The model under review builds one solid part; all positions refer to its coordinate system, in mm. A direction names the side the tool comes from. Give positions to 0.01 mm unless a question says otherwise; leave off trailing zeros. Write each loop counter-clockwise with the first axis right and the second up, starting at its lowest first coordinate (ties: lowest second). Pieces come first, ordered by that corner, then holes. Notation, with made-up numbers: (31.25, 89) - (71.25, 89) arc R19 ccw to (71.25, 123) - close; hole circle Ø5 at (34.5, 48.25). An arc over 180 degrees is marked (long way). Write item = value, one per line.
```python
from build123d import *

# Parameters (mm, degrees)
SKETCH1_W           = 171.45
SKETCH1_H           = 107.95
BOSS_EXTRUDE1_DEPTH = 3.175
BOSS_EXTRUDE2_DEPTH = 3.175
SKETCH4_W           = 50.8
SKETCH4_H           = 3.175
BOSS_EXTRUDE3_DEPTH = 19.05
CHAMFER1_SIZE       = 12.7
CHAMFER1_SIZE_2     = 10.472688289
CHAMFER1_SIZE_3     = 17.454480482
SKETCH6_W           = 88.9
SKETCH6_H           = 88.9
BOSS_EXTRUDE4_DEPTH = 3.175
BOSS_EXTRUDE7_DEPTH = 50.8


with BuildPart() as part:
    # Sketch1 → Boss-Extrude1 (new body)
    with BuildSketch(Plane(origin=(0, 0, 0), x_dir=(1, 0, 0), z_dir=(0, 1, 0))):
        Rectangle(SKETCH1_W, SKETCH1_H)
    extrude(amount=BOSS_EXTRUDE1_DEPTH)

    # Sketch2 → Boss-Extrude2 (add)
    with BuildSketch(Plane(origin=(0, 3.175, 0), x_dir=(1, 0, 0), z_dir=(0, 1, 0))):
        Polygon((-85.725, -53.975), (-82.55, -66.675), (88.9, -66.675), (85.725, -53.975), align=None)
    extrude(amount=-BOSS_EXTRUDE2_DEPTH)

    # Chamfer1
    # the kernel refuses this chamfer: 17.454480482, 12.7, 10.472688289 mm, written as the material it takes off along each edge
    with BuildSketch(Plane(origin=(88.9, 35.835373947, 66.675), x_dir=(-0.21576900793941634, 0, -0.9764444352920651), z_dir=(0, -1, 0))) as chamfer1_piece_1:
        Polygon((CHAMFER1_SIZE * 0.999621916911, -CHAMFER1_SIZE * 0.0274958766106), (CHAMFER1_SIZE_2 * 0.215769007941, -CHAMFER1_SIZE_2 * 0.976444435298), (0, 0), align=None)
    extrude(amount=68.495747894, mode=Mode.SUBTRACT)
    with BuildSketch(Plane(origin=(-82.55, 48.316843842, 66.675), x_dir=(0.9993006642791182, 0, 0.0373922768939412), z_dir=(0, -1, 0))) as chamfer1_piece_2:
        Polygon((CHAMFER1_SIZE * 0.999300664279, -CHAMFER1_SIZE * 0.0373922768939), (-CHAMFER1_SIZE_3 * 0.278641848199, -CHAMFER1_SIZE_3 * 0.960395085581), (0, 0), align=None)
    extrude(amount=93.458687684, mode=Mode.SUBTRACT)

    # Sketch6 → Boss-Extrude4 (add)
    with BuildSketch(Plane(origin=(0, 3.175, 0), x_dir=(1, 0, 0), z_dir=(0, 1, 0))):
        with Locations((0, 98.425)):
            Rectangle(SKETCH6_W, SKETCH6_H)
    extrude(amount=-BOSS_EXTRUDE4_DEPTH)



with BuildPart() as body_2:
    # Sketch4 → Boss-Extrude3 (new body)
    with BuildSketch(Plane.XZ):
        with Locations((0, 68.2625)):
            Rectangle(SKETCH4_W, SKETCH4_H)
    extrude(amount=BOSS_EXTRUDE3_DEPTH)


with BuildPart() as part_1:
    add(part.part)

    add(body_2.part)  # Boss-Extrude7 merges body 2
    # Sketch10 → Boss-Extrude7 (add)
    with BuildSketch(Plane(origin=(25.4, 0, 0), x_dir=(0, 0, -1), z_dir=(1, 0, 0))):
        with BuildLine():
            Line((-66.675, 3.175), (-66.675, 0))
            Line((-66.675, 0), (-69.85, 0))
            ThreePointArc((-69.85, 0), (-68.92006403, 2.24506403), (-66.675, 3.175))
        make_face()
    extrude(amount=-BOSS_EXTRUDE7_DEPTH)


solid = part_1.part
```
1. Take a section at B-B on y = -5.75. Give the boundary of the cut face in (x, z) (3 decimals).
Findings below:
outline = (-25.4, 66.675) - (25.4, 66.675) - (25.4, 69.85) - (-25.4, 69.85) - close
2. For line 1 (Y direction, x = 2, z = -125) (3 decimals); line 2 (Z direction, x = -7, y = -10.25) (3 decimals); line 3 (Z direction, x = -34, y = 0.5) (3 decimals), list the stretches that pass through material, from the lowest coordinate up. Write a range as from..to.
Findings below:
line_1 = 0..3.175
line_2 = 66.675..69.85
line_3 = -142.875..66.675
3. Machinability: for faces 1 (the flat face through (-1, 0, -16)), 2 (the flat face through (82.175, 1.61, 60.428)), which of the approach directions +Z, -Z, +X, -X, +Y, -Y give a long, thin tool a straight path to every point of the face, cutting with its end or side? Answer none if there is none.
Findings below:
face_1 = -Z, +X, -X, -Y
face_2 = +Z, +X, +Y, -Y
4. Insertion check: P1, Ø8, axis at x = -50.5, z = -27, coming from the -Y side; P2, Ø1, axis at y = -11, z = 69, coming from the -X side; P3, Ø2.5, axis at y = 1.5, z = -116.5, coming from the +X side; P4, Ø6, axis at x = -49.5, z = -71.5, coming from the -Y side. Each pin has a flat end and moves straight along its axis. Give the tip position at first contact, or say it passes through.
Findings below:
P1 = 0
P2 = -25.4
P3 = 44.45
P4 = through
5. Take a section at A-A on x = -19.5. Give the boundary of the cut face in (y, z) (3 decimals).
Findings below:
outline = (-19.05, 66.675) - (0, 66.675) - (0, -142.875) - (3.175, -142.875) - (3.175, 66.675) arc R3.175 ccw to (0, 69.85) - (-19.05, 69.85) - close
6. Take a section at C-C on z = -19. Give the boundary of the cut face in (x, y) (3 decimals).
Findings below:
outline = (-85.725, 0) - (85.725, 0) - (85.725, 3.175) - (-85.725, 3.175) - close
